from build123d import *

# Parameters (mm, degrees)
BOSS_EXTRUDE2_DEPTH = 1
BOSS_EXTRUDE3_DEPTH = 1
CUT_EXTRUDE3_START  = -2
CUT_EXTRUDE3_DEPTH  = 2
FILLET1_R           = 5
FILLET2_R           = 0.5
SKETCH2_R           = 1.9
BOSS_EXTRUDE4_DEPTH = 2
FILLET3_R           = 0.25


# Read off the part's stored shape, not the designer's step: Cut-Extrude3
with BuildPart() as part:
    # Sketch1 → Boss-Extrude2 (new, symmetric)
    with BuildSketch(Plane(origin=(0, 0, 0), x_dir=(1, 0, 0), z_dir=(0, 1, 0))):
        with BuildLine():
            Line((48.296291314, -12.940952255), (0, 0))
            Line((0, 0), (48.296291314, 12.940952255))
            ThreePointArc((48.296291314, 12.940952255), (50, 0), (48.296291314, -12.940952255))
        make_face()
    extrude(amount=BOSS_EXTRUDE2_DEPTH, both=True)

    # Sketch3 → Boss-Extrude3 (add)
    with BuildSketch(Plane(origin=(0, -1, 0), x_dir=(-1, 0, 0), z_dir=(0, -1, 0))):
        with BuildLine():
            Line((-38.5, -7), (-38.5, 7))
            ThreePointArc((-38.5, 7), (-38, 7.5), (-37.5, 7))
            Line((-37.5, 7), (-37.5, -7))
            ThreePointArc((-37.5, -7), (-38, -7.5), (-38.5, -7))
        make_face()
    extrude(amount=BOSS_EXTRUDE3_DEPTH)

    # Cut-Extrude3 outline → Cut-Extrude3 (cut)
    with BuildSketch(Plane(origin=(0, 1, 0), x_dir=(1, 0, 0), z_dir=(0, 1, 0)).offset(CUT_EXTRUDE3_START)):
        with BuildLine():
            ThreePointArc((39.129720832, 10.484777097), (44.969397941, 4.720942194), (49.96810207, -1.785714286))
            ThreePointArc((49.96810207, -1.785714286), (49.680896013, 5.639908806), (48.296291314, 12.940952255))
            Line((48.296291314, 12.940952255), (39.129720832, 10.484777097))
        make_face()
    extrude(amount=CUT_EXTRUDE3_DEPTH, mode=Mode.SUBTRACT)

    # Fillet1
    fillet1_edges = [part.edges().sort_by_distance(p)[0] for p in [
        (39.129720832, 0, -10.484777097),
        (49.96810207, 0, 1.785714286),
        (48.296291314, 0, 12.940952255),
    ]]
    fillet(fillet1_edges, radius=FILLET1_R)

    # Fillet2
    fillet2_edges = [part.edges().sort_by_distance(p)[0] for p in [
        (18.252899917, -1, -4.890849792),
        (18.252899917, 1, -4.890849792),
        (45.320316883, -1, -4.32008237),
        (49.692435611, -1, 5.537313704),
        (21.598758088, -1, 5.787369787),
        (47.228674266, -1, 10.929424828),
        (49.700770587, -1, 1.869330184),
        (39.027043508, -1, -9.799142423),
        (45.320316883, 1, -4.32008237),
        (21.598758088, 1, 5.787369787),
        (49.692435611, 1, 5.537313704),
        (47.228674266, 1, 10.929424828),
        (49.700770587, 1, 1.869330184),
        (39.027043508, 1, -9.799142423),
    ]]
    fillet(fillet2_edges, radius=FILLET2_R)

    # Sketch2 → Boss-Extrude4 (add)
    with BuildSketch(Plane(origin=(0, 1, 0), x_dir=(1, 0, 0), z_dir=(0, 1, 0))):
        with Locations(Location((42.5, 0, 0), (0, 0, 90))):
            Circle(SKETCH2_R)
    extrude(amount=BOSS_EXTRUDE4_DEPTH)

    # Fillet3
    fillet3_edges = [part.edges().sort_by_distance(p)[0] for p in [
        (42.5, 3, 1.9),
    ]]
    fillet(fillet3_edges, radius=FILLET3_R)


solid = part.part
Source: CAD feature listing. Evaluate the final solid. Frame: model axes, mm. A direction names the side the tool comes from. Give positions to 0.01 mm unless a question says otherwise; leave off trailing zeros. Order: outer loops, then holes, each group sorted by start corner. A loop starts at its lowest first (then second) coordinate and runs counter-clockwise, first axis right, second up. Notation, with made-up numbers: (16.5, 8) -> (47.5, 8) arc R16 cw to (47.5, 39) -> close; hole circle Ø9 at (8.5, -16). An arc over 180 degrees is marked (long way). Write item = value, one per line.
Q1. Material intervals for line 1 (X direction, y = -1.6, z = 1.25); line 2 (Y direction, x = 18.5, z = 2.25); line 3 (Y direction, x = 29.5, z = 7.75), sorted ascending. Write a range as from..to.
Data:
line_1 = 37.5..38.5
line_2 = -1..1
line_3 = -0.86..0.86
Q2. Set-up query: faces 1 (the face through (44.355, 1.863, 0.412)), 2 (the face through (37.5, -1.5, -0.1)), 3 (the face through (38, -1.5, -7.5)), 4 (the face through (38.5, -1.5, 0.1)). Return all of +Z, -Z, +X, -X, +Y, -Y with unobstructed straight access to the full face (end or side cutting, diameter ignored); none if empty.
Data:
face_1 = +Y
face_2 = +Z, -Z, -X, -Y
face_3 = -Z, -Y
face_4 = +Z, -Z, +X, -Y
Q3. Cut plane A-A, the plane y = 2.05. Output: boundary loops of the cut face in (x, z).
Data:
outline = circle Ø3.8 at (42.5, 0)
Q4. Pin query (flat end, axial travel): pin 1 (5 mm diameter, centred on x = 24.5, z = 5, fed in from +Y); pin 2 (2 mm diameter, centred on x = 19, y = 0, fed in from -Z); pin 3 (0.8 mm diameter, centred on y = -1.5, z = -3, fed in from +X). Return the tip coordinate at first contact, or that it passes through.
Data:
pin_1 = 1
pin_2 = -5.36
pin_3 = 38.5
